Print and shaded views of the part. All mm, measured from the part's lowest x, y and z. Give positions to 0.01 mm unless a question says otherwise; leave off trailing zeros. Order: outer loops, then holes, each group sorted by start corner. A loop starts at its lowest first (then second) coordinate and runs counter-clockwise, first axis right, second up. Notation, with made-up numbers: (-3.75, 46) - (27.25, 46) arc R18 cw to (27.25, 52) - close; hole circle Ø1 at (65, -32). An arc over 180 degrees is marked (long way). Answer in a Markdown table with one row per item.
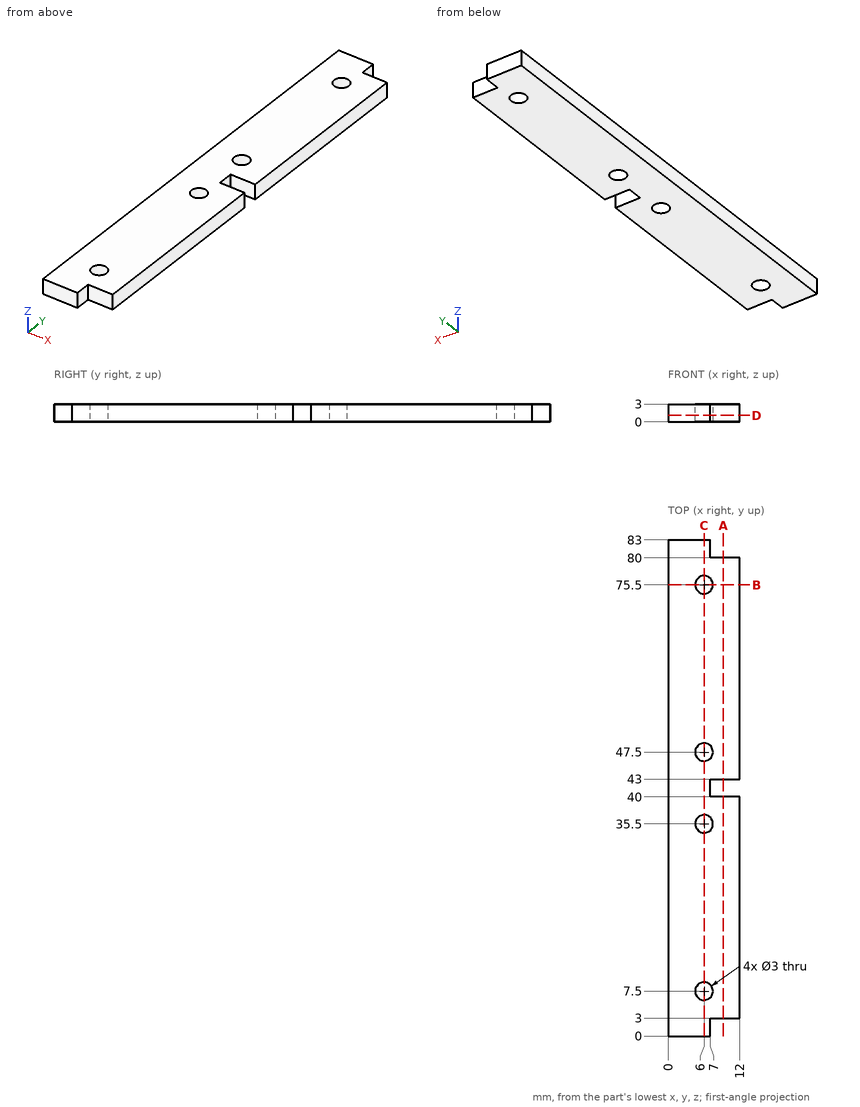
1. Probe line 1 (Y direction, x = 6, z = 0.65); line 2 (X direction, y = 75.5, z = 1.3); line 3 (Y direction, x = 8, z = 2.5). List the from-to ranges inside material, lowest first.
Check result:
| item | result |
|---|---|
| line 1 | y = 0 to 6, 9 to 34, 37 to 46, 49 to 74, 77 to 83 |
| line 2 | x = 0 to 4.5, 7.5 to 12 |
| line 3 | y = 3 to 40, 43 to 80 |
2. Drop flat-ended pins along their axis: P1, Ø2.5, axis at x = 6, y = 7.5, coming from the -Z side; P2, Ø1.5, axis at y = 1, z = 2, coming from the +X side; P3, Ø1, axis at x = 9, z = 1.5, coming from the +Y side; P4, Ø1.5, axis at x = 9.5, z = 1, coming from the -Y side. Give the stop position or say it passes through.
Check result:
| item | result |
|---|---|
| P1 | passes through |
| P2 | stops at x = 7 |
| P3 | stops at y = 80 |
| P4 | stops at y = 3 |
3. Cut at C-C on x = 6. Write the cut outline in (y, z), and give its area (3 significant figures).
Check result:
| item | result |
|---|---|
| outline | (0, 0) - (6, 0) - (6, 3) - (0, 3) - close; (9, 0) - (34, 0) - (34, 3) - (9, 3) - close; (37, 0) - (46, 0) - (46, 3) - (37, 3) - close; (49, 0) - (74, 0) - (74, 3) - (49, 3) - close; (77, 0) - (83, 0) - (83, 3) - (77, 3) - close |
| area | 213 mm² |
4. Cut at B-B on y = 75.5. Write the cut outline in (x, z).
Check result:
| item | result |
|---|---|
| outline | (0, 0) - (4.5, 0) - (4.5, 3) - (0, 3) - close; (7.5, 0) - (12, 0) - (12, 3) - (7.5, 3) - close |
5. Cut at A-A on x = 9.25. Write the cut outline in (y, z), and give its area (3 significant figures).
Check result:
| item | result |
|---|---|
| outline | (3, 0) - (40, 0) - (40, 3) - (3, 3) - close; (43, 0) - (80, 0) - (80, 3) - (43, 3) - close |
| area | 222 mm² |
6. Cut at D-D on z = 1.1. Write the cut outline in (x, y), and give its area (3 significant figures).
Check result:
| item | result |
|---|---|
| outline | (0, 0) - (7, 0) - (7, 3) - (12, 3) - (12, 40) - (7, 40) - (7, 43) - (12, 43) - (12, 80) - (7, 80) - (7, 83) - (0, 83) - close; hole circle Ø3 at (6, 7.5); hole circle Ø3 at (6, 35.5); hole circle Ø3 at (6, 47.5); hole circle Ø3 at (6, 75.5) |
| area | 923 mm² |
